Can you work these out from the model? Positions are in its coordinate system, mm. Round coordinates to 2 decimals unless told otherwise and drop trailing zeros. One line per item, written item: value.
```python
from build123d import *

# Parameters (mm, degrees)
F0_W     = 479.425
F0_H     = 66.675
F1_DEPTH = 3.175
F2_W     = 3.175
F2_H     = 9.525
F3_DEPTH = 3.176
F4_W     = 9.525
F4_H     = 3.175
F5_DEPTH = 3.176
F6_R     = 1.5875
F7_DEPTH = 3.176


with BuildPart() as f1:
    # F0 (on Front) → F1 (new body)
    with BuildSketch(Plane.XZ):
        Rectangle(F0_W, F0_H)
    extrude(amount=F1_DEPTH)

    # F2 (on face) → F3 (cut, through all)
    with BuildSketch(Plane.XZ.offset(3.175)):
        with Locations((-238.125, -28.575)):
            Rectangle(F2_W, F2_H)
        with Locations((-238.125, -9.525)):
            Rectangle(F2_W, F2_H)
        with Locations((-238.125, 9.525)):
            Rectangle(F2_W, F2_H)
        with Locations((-238.125, 28.575)):
            Rectangle(F2_W, F2_H)
        with Locations((-158.75, -28.575)):
            Rectangle(F2_W, F2_H)
        with Locations((-158.75, -9.525)):
            Rectangle(F2_W, F2_H)
        with Locations((-158.75, 9.525)):
            Rectangle(F2_W, F2_H)
        with Locations((-158.75, 28.575)):
            Rectangle(F2_W, F2_H)
        with Locations((-79.375, -28.575)):
            Rectangle(F2_W, F2_H)
        with Locations((-79.375, -9.525)):
            Rectangle(F2_W, F2_H)
        with Locations((-79.375, 9.525)):
            Rectangle(F2_W, F2_H)
        with Locations((-79.375, 28.575)):
            Rectangle(F2_W, F2_H)
        with Locations((0, -28.575)):
            Rectangle(F2_W, F2_H)
        with Locations((0, -9.525)):
            Rectangle(F2_W, F2_H)
        with Locations((0, 9.525)):
            Rectangle(F2_W, F2_H)
        with Locations((0, 28.575)):
            Rectangle(F2_W, F2_H)
        with Locations((79.375, -28.575)):
            Rectangle(F2_W, F2_H)
        with Locations((79.375, -9.525)):
            Rectangle(F2_W, F2_H)
        with Locations((79.375, 9.525)):
            Rectangle(F2_W, F2_H)
        with Locations((79.375, 28.575)):
            Rectangle(F2_W, F2_H)
        with Locations((158.75, -28.575)):
            Rectangle(F2_W, F2_H)
        with Locations((158.75, -9.525)):
            Rectangle(F2_W, F2_H)
        with Locations((158.75, 9.525)):
            Rectangle(F2_W, F2_H)
        with Locations((158.75, 28.575)):
            Rectangle(F2_W, F2_H)
        with Locations((238.125, -28.575)):
            Rectangle(F2_W, F2_H)
        with Locations((238.125, -9.525)):
            Rectangle(F2_W, F2_H)
        with Locations((238.125, 9.525)):
            Rectangle(F2_W, F2_H)
        with Locations((238.125, 28.575)):
            Rectangle(F2_W, F2_H)
    extrude(amount=-F3_DEPTH, mode=Mode.SUBTRACT)

    # F4 (on face) → F5 (cut, through all)
    with BuildSketch(Plane.XZ.offset(3.175)):
        with Locations((-219.075, -31.75)):
            Rectangle(F4_W, F4_H)
        with Locations((-198.4375, -31.75)):
            Rectangle(F4_W, F4_H)
        with Locations((-177.8, -31.75)):
            Rectangle(F4_W, F4_H)
        with Locations((-139.7, -31.75)):
            Rectangle(F4_W, F4_H)
        with Locations((-119.0625, -31.75)):
            Rectangle(F4_W, F4_H)
        with Locations((-98.425, -31.75)):
            Rectangle(F4_W, F4_H)
        with Locations((-60.325, -31.75)):
            Rectangle(F4_W, F4_H)
        with Locations((-39.6875, -31.75)):
            Rectangle(F4_W, F4_H)
        with Locations((-19.05, -31.75)):
            Rectangle(F4_W, F4_H)
        with Locations((19.05, -31.75)):
            Rectangle(F4_W, F4_H)
        with Locations((39.6875, -31.75)):
            Rectangle(F4_W, F4_H)
        with Locations((60.325, -31.75)):
            Rectangle(F4_W, F4_H)
        with Locations((98.425, -31.75)):
            Rectangle(F4_W, F4_H)
        with Locations((119.0625, -31.75)):
            Rectangle(F4_W, F4_H)
        with Locations((139.7, -31.75)):
            Rectangle(F4_W, F4_H)
        with Locations((177.8, -31.75)):
            Rectangle(F4_W, F4_H)
        with Locations((198.4375, -31.75)):
            Rectangle(F4_W, F4_H)
        with Locations((219.075, -31.75)):
            Rectangle(F4_W, F4_H)
    extrude(amount=-F5_DEPTH, mode=Mode.SUBTRACT)

    # F6 (on face) → F7 (cut, through all)
    with BuildSketch(Plane.XZ.offset(3.175)):
        with Locations((-39.6875, 0)):
            Circle(F6_R)
        with Locations((39.6875, 0)):
            Circle(F6_R)
    extrude(amount=-F7_DEPTH, mode=Mode.SUBTRACT)


solid = f1.part
```
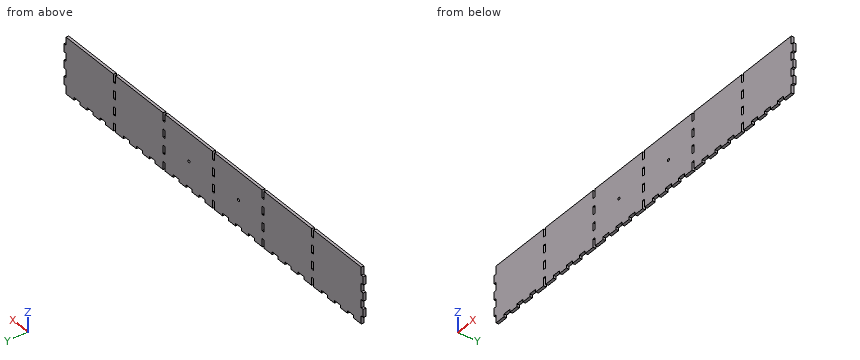
Q1. Please list where these lines run through material, in increasing order: line 1 along X through (y, z) = (-1.9, -25.5); line 2 along Z through (x, y) = (135, -1.3); line 3 along Z through (x, y) = (-41, -0.6).
Answers below:
line 1: -236.54 to -160.34, -157.16 to -80.96, -77.79 to -1.59, 1.59 to 77.79, 80.96 to 157.16, 160.34 to 236.54
line 2: -30.16 to 33.34
line 3: -30.16 to -0.89, 0.89 to 33.34
Q2. I want a section at A-A on y = -1.3. Give the number of separate pieces and of enclosed holes in the cut face, plus the area to 3 significant figures.
Answers below:
separate pieces: 1
enclosed holes: 12
area: 30,600 mm^2
Q3. Will these pins go through, and if not, where does the flat tip stop? pin 1 Ø1 at (x, y) = (238, -1) entering from -Z; pin 2 Ø1.6 at (x, y) = (177, -1.5) entering from -Z; pin 3 Ø1 at (y, z) = (-1, -8.5) entering from +X.
Answers below:
pin 1: z = -23.81
pin 2: z = -30.16
pin 3: x = 236.54
